from build123d import *

# Parameters (mm, degrees)
F0_R          = 30
F0_R_2        = 27
F1_DEPTH      = 135
F1_DEPTH_BACK = 25
F0_R_3        = 14.7
F2_DEPTH      = 25
F0_R_4        = 7.5
F3_DEPTH      = 5
F5_DEPTH      = 20
F5_DEPTH_BACK = 5
F7_DEPTH      = 20


with BuildPart() as f1:
    # F0 (on Front) → F1 (new body, two sides)
    with BuildSketch(Plane.XZ) as f1_sk:
        Circle(F0_R)
        Circle(F0_R_2, mode=Mode.SUBTRACT)
    extrude(amount=-F1_DEPTH)
    extrude(f1_sk.sketch, amount=F1_DEPTH_BACK)

    # F0 (on Front) → F2 (join)
    with BuildSketch(Plane.XZ):
        Circle(F0_R_2)
        Circle(F0_R_3, mode=Mode.SUBTRACT)
    extrude(amount=-F2_DEPTH)

    # F0 (on Front) → F3 (join)
    with BuildSketch(Plane.XZ):
        Circle(F0_R_3)
        Circle(F0_R_4, mode=Mode.SUBTRACT)
    extrude(amount=-F3_DEPTH)

    # F4 (on Front) → F5 (join, two sides)
    with BuildSketch(Plane.XZ) as f5_sk:
        with BuildLine():
            Line((-25, 35), (-25, 16.5831239518))
            ThreePointArc((-25, 16.5831239518), (0, 30), (25, 16.5831239518))
            Line((25, 16.5831239518), (25, 35))
            Line((25, 35), (-25, 35))
        make_face()
    extrude(amount=F5_DEPTH)
    extrude(f5_sk.sketch, amount=-F5_DEPTH_BACK)

    # F6 (on face) → F7 (cut)
    with BuildSketch(Plane.XY.offset(35)):
        Polygon((0, 0), (-17.5, 0), (-17.5, -15), (17.5, -15), (17.5, 0), align=None)
    extrude(amount=-F7_DEPTH, mode=Mode.SUBTRACT)


solid = f1.part
The listing builds one solid part. Answer for the finished solid, in the listing's coordinates (mm). A direction names the side the tool comes from. Give positions to 0.01 mm unless a question says otherwise; leave off trailing zeros. Write each loop counter-clockwise with the first axis right and the second up, starting at its lowest first coordinate (ties: lowest second). Pieces come first, ordered by that corner, then holes.
Item 1: Section D-D, the plane x = -10.5 is taken. Write down the section's boundary in (y, z).
Item 2: Which of the six approach directions +Z, -Z, +X, -X, +Y, -Y give full straight-line access (tool end or side, diameter ignored) to faces 1 (the cylindrical face through (-5.85, -12.32, -26.36)), 2 (the flat face through (0, -15, 29)), 3 (the flat face through (-25, -8, 26)), 4 (the flat face through (25, -8, 26)), 5 (the cylindrical face through (-5.85, 79.23, -26.36))?
Item 3: Determine the mould class of faces 6 (the flat face through (6, 5, -6)), 7 (the cylindrical face through (-6.503, 56.12, -29.287)), 8 (the flat face through (17.5, -8, 28)), 9 (the flat face through (12, 25, -12)) for opening direction Z: released by +Z, released by -Z, zero draft, split by the parting line, or undercut.
Item 4: Section C-C, the plane y = -10 is taken. Write down the section's boundary in (x, z), plus the area to 3 significant figures.
Item 5: Section A-A, the plane z = 0 is taken. Write down the section's boundary in (x, y).
Item 6: Find the intervals of material crossed by line 1 along Y through (x, z) = (2, 30); line 2 along Y through (x, z) = (-18, 2.5); line 3 along Z through (x, y) = (0, 95), in increasing order.
Item 7: Section B-B, the plane x = 0 is taken. Write down the section's boundary in (y, z), plus the area to 3 significant figures.
Item 8: Flat-ended cylindrical pins translate along their axes: P1, Ø3, axis at x = -17, y = 115, coming from the +Z side; P2, Ø16, axis at x = -1.5, z = -10.5, coming from the +Y side; P3, Ø16, axis at y = -10.5, z = 24.5, coming from the -X side. Find the tip coordinate at first contact, or state that the pin passes through.
Completed:
1. outline: (-25, -28.1) - (135, -28.1) - (135, -24.87) - (25, -24.87) - (25, -10.29) - (5, -10.29) - (5, 10.29) - (25, 10.29) - (25, 24.87) - (135, 24.87) - (135, 28.1) - (5, 28.1) - (5, 35) - (0, 35) - (0, -24.87) - (-25, -24.87) - close; (-25, 24.87) - (-15, 24.87) - (-15, 35) - (-20, 35) - (-20, 28.1) - (-25, 28.1) - close
2. face 1: -Y
2. face 2: +Z
2. face 3: +Z, -X, +Y, -Y
2. face 4: +Z, +X, +Y, -Y
2. face 5: +Y
3. face 6: undercut
3. face 7: split by the parting line
3. face 8: zero draft
3. face 9: undercut
4. outline: (-25, 16.58) arc R30 ccw (long way) to (25, 16.58) - (25, 35) - (17.5, 35) - (17.5, 20.56) arc R27 cw (long way) to (-17.5, 20.56) - (-17.5, 35) - (-25, 35) - close
4. area: 635 mm2
5. outline: (-30, -25) - (-27, -25) - (-27, 0) - (-7.5, 0) - (-7.5, 5) - (-14.7, 5) - (-14.7, 25) - (-27, 25) - (-27, 135) - (-30, 135) - close; (7.5, 0) - (27, 0) - (27, -25) - (30, -25) - (30, 135) - (27, 135) - (27, 25) - (14.7, 25) - (14.7, 5) - (7.5, 5) - close
6. line 1: y = -20 to -15, 0 to 5
6. line 2: y = 0 to 25
6. line 3: z = -30 to -27, 27 to 30
7. outline: (-25, -30) - (135, -30) - (135, -27) - (25, -27) - (25, -14.7) - (5, -14.7) - (5, -7.5) - (0, -7.5) - (0, -27) - (-25, -27) - close; (-25, 27) - (-15, 27) - (-15, 35) - (-20, 35) - (-20, 30) - (-25, 30) - close; (0, 7.5) - (5, 7.5) - (5, 14.7) - (25, 14.7) - (25, 27) - (135, 27) - (135, 30) - (5, 30) - (5, 35) - (0, 35) - close
7. area: 1,650 mm2
8. P1: stops at z = 25.69
8. P2: stops at y = 25
8. P3: stops at x = -25.05
